Model file for the job. Use its own axes, mm. Face numbers are marked on the shaded views. Coordinates: 2 decimals unless noted, no trailing zeros. Write each loop counter-clockwise with the first axis right and the second up, starting at its lowest first coordinate (ties: lowest second). Pieces come first, ordered by that corner, then holes.
Q1. Band-saw the part on D-D, the plane x = 4. Write the cut outline in (y, z), plus the area to 3 significant figures.
Q2. Band-saw the part on C-C, the plane y = 0. Write the cut outline in (x, z) (3 decimals).
Q3. Band-saw the part on B-B, the plane x = 0. Write the cut outline in (y, z) (3 decimals), plus the area to 3 significant figures.
Q4. Pin check, flat tips, straight feed: P1, Ø1, axis at x = -2.5, y = 3, coming from the -Z side; P2, Ø1, axis at x = 0.5, z = 14.5, coming from the -Y side; P3, Ø5, axis at x = 4.5, z = 22, coming from the +Y side; P4, Ø1.8, axis at x = 0.5, y = -1.5, coming from the -Z side. Stop position of each tip, or through.
Q5. Pull direction X, two halves, no side cores. Call the marked faces 1, 2 and 3: released by +X, released by -X, zero draft, split by the parting line, or undercut.
Q6. Drill centre lines: probe 1 along Y at (x, z) = (0, 14.5) (3 decimals); probe 2 along Y at (x, z) = (-0.5, 15); probe 3 along X at (y, z) = (8, 8.5). Where is each one in solid material? Low to high.
Q7. Band-saw the part on A-A, the plane x = -2.25. Write the cut outline in (y, z).
from build123d import *

# Parameters (mm, degrees)
EXTRUDE1_DEPTH      = 25
EXTRUDE1_DEPTH_BACK = 0.001
SKETCH3_R           = 1.5
CUT_EXTRUDE1_DEPTH  = 28.804066937
SKETCH5_R           = 4.335
CUT_EXTRUDE2_DEPTH  = 24


with BuildPart() as part:
    # Sketch1 → Extrude1 (new, two sides: drawn at the far end of the back side and taken through both)
    with BuildSketch(Plane.XY.offset(-EXTRUDE1_DEPTH_BACK)):
        with BuildLine():
            ThreePointArc((5.394294709, 9.281673418), (7.083207262, 0), (5.394294709, -9.281673418))
            ThreePointArc((5.394294709, -9.281673418), (0.839593343, -9.873480825), (-3.625620963, -8.797654747))
            ThreePointArc((-3.625620963, -8.797654747), (-3.857898862, -8.166383103), (-3.57576768, -7.555761366))
            ThreePointArc((-3.57576768, -7.555761366), (-0.970954643, 0.05080099), (-3.638712866, 7.635516404))
            ThreePointArc((-3.638712866, 7.635516404), (-3.831936153, 8.239573474), (-3.57576768, 8.819744049))
            ThreePointArc((-3.57576768, 8.819744049), (0.866819678, 9.874912356), (5.394294709, 9.281673418))
        make_face()
    extrude(amount=EXTRUDE1_DEPTH + EXTRUDE1_DEPTH_BACK)

    # Sketch3 → Cut-Extrude1 (cut, through all)
    with BuildSketch(Plane.XY.offset(25)):
        with Locations((0, 6.715)):
            Circle(SKETCH3_R)
        with Locations(Location((0, -6.715, 0), (0, 0, 180))):
            Circle(SKETCH3_R)
    extrude(amount=-CUT_EXTRUDE1_DEPTH, mode=Mode.SUBTRACT)

    # Sketch5 → Cut-Extrude2 (cut)
    with BuildSketch(Plane(origin=(0, 0, -0.001), x_dir=(-1, 0, 0), z_dir=(0, 0, -1))):
        Circle(SKETCH5_R)
    extrude(amount=-CUT_EXTRUDE2_DEPTH, mode=Mode.SUBTRACT)


solid = part.part
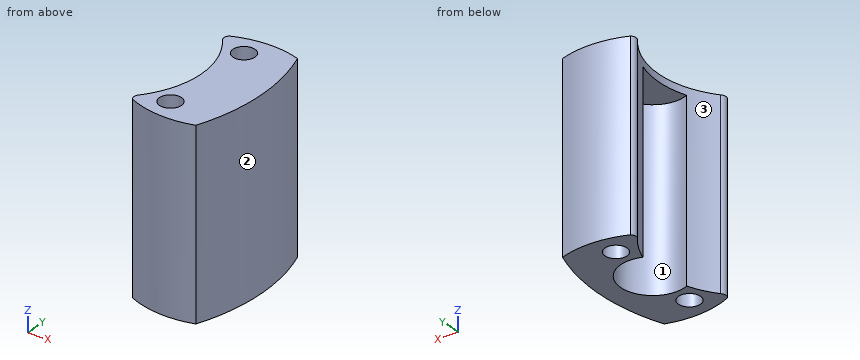
Answer sheet:
1. outline: (-9.65, 0) - (-1.67, 0) - (-1.67, 24) - (1.67, 24) - (1.67, 0) - (9.65, 0) - (9.65, 25) - (-9.65, 25) - close
1. area: 402 mm2
2. outline: (-0.971, 23.999) - (4.335, 23.999) - (4.335, -0.001) - (7.083, -0.001) - (7.083, 25) - (-0.971, 25) - close
3. outline: (-9.8, -0.001) - (-8.215, -0.001) - (-8.215, 25) - (-9.8, 25) - close; (-5.215, -0.001) - (-4.335, -0.001) - (-4.335, 23.999) - (4.335, 23.999) - (4.335, -0.001) - (5.215, -0.001) - (5.215, 25) - (-5.215, 25) - close; (8.215, -0.001) - (9.8, -0.001) - (9.8, 25) - (8.215, 25) - close
3. area: 132 mm2
4. P1: passes through
4. P2: stops at y = -9.88
4. P3: stops at y = 9.88
4. P4: stops at z = 24
5. face 1: undercut
5. face 2: released by +X
5. face 3: released by -X
6. probe 1: y = -9.8 to -8.215, -5.215 to -4.335, 4.335 to 5.215, 8.215 to 9.8
6. probe 2: y = -9.73 to -8.13, -5.3 to -4.31, 4.31 to 5.3, 8.13 to 9.73
6. probe 3: x = -3.81 to -0.77, 0.77 to 5.84
7. outline: (-9.32, 0) - (-5.45, 0) - (-5.45, 25) - (-9.32, 25) - close; (5.45, 0) - (9.32, 0) - (9.32, 25) - (5.45, 25) - close
